Can you work these out from the model? Positions are in its coordinate system, mm. Coordinates: 2 decimals unless noted, no trailing zeros. Order: outer loops, then holes, each group sorted by start corner. A loop starts at its lowest first (then second) coordinate and runs counter-clockwise, first axis right, second up.
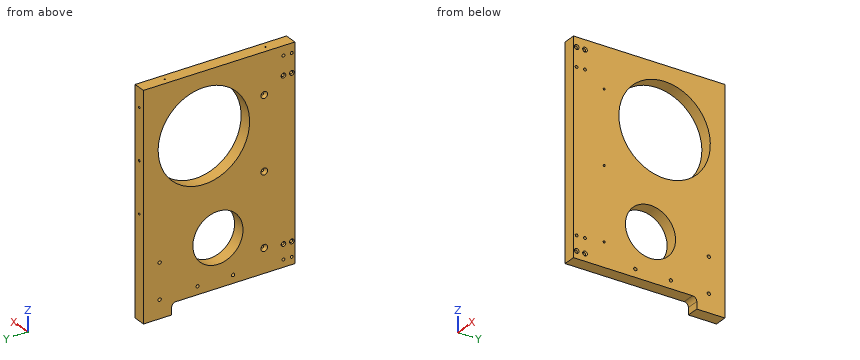
```python
from build123d import *

# Parameters (mm, degrees)
SKETCH1_W                                         = 19.05
SKETCH1_H                                         = 230.1875
BOSS_EXTRUDE1_DEPTH                               = 342.9
SKETCH2_W                                         = 19.05
SKETCH2_H                                         = 156.880836743
CUT_EXTRUDE1_DEPTH                                = 8.255
F_15_64_0_23438_DIAMETER_HOLE3_D                  = 5.953252
F_15_64_0_23438_DIAMETER_HOLE3_DEPTH              = 12.7
F_15_64_0_23438_DIAMETER_HOLE3_TIP                = 1.788537341
F_5_64_0_07813_DIAMETER_HOLE1_D                   = 3.175
F_5_64_0_07813_DIAMETER_HOLE1_DEPTH               = 38.1
F_5_64_0_07813_DIAMETER_HOLE1_CSINK_D             = 10.16
F_5_64_0_07813_DIAMETER_HOLE1_CSINK_ANGLE         = 82
F_5_64_0_07813_DIAMETER_HOLE1_TIP                 = 0.953866233
F_5_64_0_07813_DIAMETER_HOLE2_D                   = 1.984502
F_5_64_0_07813_DIAMETER_HOLE2_DEPTH               = 38.1
F_5_64_0_07813_DIAMETER_HOLE2_CSINK_D             = 10.16
F_5_64_0_07813_DIAMETER_HOLE2_CSINK_ANGLE         = 82
F_5_64_0_07813_DIAMETER_HOLE2_TIP                 = 0.59620455
F_1_8_0_125_DIAMETER_HOLE1_D                      = 3.175
F_1_8_0_125_DIAMETER_HOLE1_DEPTH                  = 19.05
F_1_8_0_125_DIAMETER_HOLE1_CSINK_D                = 10.16
F_1_8_0_125_DIAMETER_HOLE1_CSINK_ANGLE            = 90
F_8_CLEARANCE_HOLE1_D                             = 4.9149
F_8_CLEARANCE_HOLE1_DEPTH                         = 19.05
CSK_FOR_6_FLAT_HEAD_MACHINE_SCREW_100_D           = 4.3053
CSK_FOR_6_FLAT_HEAD_MACHINE_SCREW_100_DEPTH       = 19.05
CSK_FOR_6_FLAT_HEAD_MACHINE_SCREW_100_CSINK_D     = 7.0866
CSK_FOR_6_FLAT_HEAD_MACHINE_SCREW_100_CSINK_ANGLE = 82
CSK_FOR_6_FLAT_HEAD_MACHINE_SCREW1_D              = 4.3053
CSK_FOR_6_FLAT_HEAD_MACHINE_SCREW1_DEPTH          = 19.05
CSK_FOR_6_FLAT_HEAD_MACHINE_SCREW1_CSINK_D        = 7.0866
CSK_FOR_6_FLAT_HEAD_MACHINE_SCREW1_CSINK_ANGLE    = 82
CUT_EXTRUDE3_REACH                                = 21.05
SKETCH22_W                                        = 25.4
SKETCH22_H                                        = 187.3885
FILLET1_R                                         = 6.35
F_8_CLEARANCE_HOLE2_D                             = 4.9149
CUT_EXTRUDE2_REACH                                = 21.05
SKETCH17_R                                        = 69.5325
SKETCH17_R_2                                      = 38.1


with BuildPart() as part:
    # Sketch1 → Boss-Extrude1 (new body)
    with BuildSketch(Plane.XY):
        with Locations((-281.19705, -118.26875)):
            Rectangle(SKETCH1_W, SKETCH1_H)
    extrude(amount=BOSS_EXTRUDE1_DEPTH)

    # Sketch2 → Cut-Extrude1 (cut)
    with BuildSketch(Plane.XY):
        with Locations((-281.19705, -81.615418372)):
            Rectangle(SKETCH2_W, SKETCH2_H)
    extrude(amount=CUT_EXTRUDE1_DEPTH, mode=Mode.SUBTRACT)

    # 15/64 (0.23438) Diameter Hole3
    with Locations(Plane(origin=(-182.40375, 1936.853954382, -6.35), x_dir=(1, 0, 0), z_dir=(0, 0, -1))):
        with Locations((-262.8265, 2051.088542934), (-262.8265, 2014.068680083), (-262.8265, 1977.048817232), (-98.7933, 2115.959791125), (-98.7933, 2151.166454382)):
            Hole(F_15_64_0_23438_DIAMETER_HOLE3_D / 2, depth=F_15_64_0_23438_DIAMETER_HOLE3_DEPTH)
            with Locations((0, 0, -(F_15_64_0_23438_DIAMETER_HOLE3_DEPTH + F_15_64_0_23438_DIAMETER_HOLE3_TIP / 2))):  # 118° drill point
                Cone(0, F_15_64_0_23438_DIAMETER_HOLE3_D / 2, F_15_64_0_23438_DIAMETER_HOLE3_TIP, mode=Mode.SUBTRACT)

    # 5/64 (0.07813) Diameter Hole1
    with Locations(Plane(origin=(-182.40375, 15.875, 6471.459863233), x_dir=(1, 0, 0), z_dir=(0, 1, 0))):
        with Locations((-262.8265, 6157.452363233), (-98.7933, 6157.452363233), (-262.8265, 6233.652363233), (-98.7933, 6233.652363233), (-262.8265, 6309.852363233), (-98.7933, 6309.852363233), (-267.97, 6119.034863233), (-115.57, 6119.034863233), (-1.27, 6119.034863233), (113.03, 6119.034863233), (265.43, 6119.034863233), (96.2533, 6309.852363233), (260.2865, 6309.852363233), (96.2533, 6233.652363233), (260.2865, 6233.652363233), (96.2533, 6157.452363233), (260.2865, 6157.452363233)):
            CounterSinkHole(F_5_64_0_07813_DIAMETER_HOLE1_D / 2, F_5_64_0_07813_DIAMETER_HOLE1_CSINK_D / 2, depth=F_5_64_0_07813_DIAMETER_HOLE1_DEPTH, counter_sink_angle=F_5_64_0_07813_DIAMETER_HOLE1_CSINK_ANGLE)
            with Locations((0, 0, -(F_5_64_0_07813_DIAMETER_HOLE1_DEPTH + F_5_64_0_07813_DIAMETER_HOLE1_TIP / 2))):  # 118° drill point
                Cone(0, F_5_64_0_07813_DIAMETER_HOLE1_D / 2, F_5_64_0_07813_DIAMETER_HOLE1_TIP, mode=Mode.SUBTRACT)

    # 5/64 (0.07813) Diameter Hole2
    with Locations(Plane(origin=(-182.40375, 1936.853954382, 361.95), x_dir=(-1, 0, 0), z_dir=(0, 0, 1))):
        with Locations((-263.392416364, 1965.434682144), (262.8265, 1964.708862949), (262.8265, 2063.428497217), (98.7933, 2131.851871048), (98.7933, 1978.393537715), (53.56098, 2123.543954382), (-53.56098, 2123.543954382), (-99.322089753, 1978.666800322), (-98.898757225, 2132.124549748), (-263.120086856, 2064.153940785)):
            CounterSinkHole(F_5_64_0_07813_DIAMETER_HOLE2_D / 2, F_5_64_0_07813_DIAMETER_HOLE2_CSINK_D / 2, depth=F_5_64_0_07813_DIAMETER_HOLE2_DEPTH, counter_sink_angle=F_5_64_0_07813_DIAMETER_HOLE2_CSINK_ANGLE)
            with Locations((0, 0, -(F_5_64_0_07813_DIAMETER_HOLE2_DEPTH + F_5_64_0_07813_DIAMETER_HOLE2_TIP / 2))):  # 118° drill point
                Cone(0, F_5_64_0_07813_DIAMETER_HOLE2_D / 2, F_5_64_0_07813_DIAMETER_HOLE2_TIP, mode=Mode.SUBTRACT)

    # 1/8 (0.125) Diameter Hole1
    with Locations(Plane.ZY.offset(290.72205)):
        with Locations((61.9125, -186.69), (280.9875, -186.69), (171.45, -186.69)):
            CounterSinkHole(F_1_8_0_125_DIAMETER_HOLE1_D / 2, F_1_8_0_125_DIAMETER_HOLE1_CSINK_D / 2, depth=F_1_8_0_125_DIAMETER_HOLE1_DEPTH, counter_sink_angle=F_1_8_0_125_DIAMETER_HOLE1_CSINK_ANGLE)

    # #8 Clearance Hole1
    with Locations(Plane(origin=(-271.67205, 0, 0), x_dir=(0, 0, -1), z_dir=(1, 0, 0))):
        with Locations((-88.9, -27.7495), (-35.8275, -27.7495)):
            Hole(F_8_CLEARANCE_HOLE1_D / 2, depth=F_8_CLEARANCE_HOLE1_DEPTH)

    # CSK for #6 Flat Head Machine Screw (100)1
    with Locations(Plane(origin=(-271.67205, 0, 0), x_dir=(0, 0, -1), z_dir=(1, 0, 0))):
        with Locations((-36.5125, -215.9), (-36.5125, -228.6), (-328.6125, -215.9), (-328.6125, -228.6)):
            CounterSinkHole(CSK_FOR_6_FLAT_HEAD_MACHINE_SCREW_100_D / 2, CSK_FOR_6_FLAT_HEAD_MACHINE_SCREW_100_CSINK_D / 2, depth=CSK_FOR_6_FLAT_HEAD_MACHINE_SCREW_100_DEPTH, counter_sink_angle=CSK_FOR_6_FLAT_HEAD_MACHINE_SCREW_100_CSINK_ANGLE)

    # CSK for #6 Flat Head Machine Screw1
    with Locations(Plane.ZY.offset(290.72205)):
        with Locations((58.7375, -228.6), (58.7375, -215.9), (300.0375, -228.6), (300.0375, -215.9)):
            CounterSinkHole(CSK_FOR_6_FLAT_HEAD_MACHINE_SCREW1_D / 2, CSK_FOR_6_FLAT_HEAD_MACHINE_SCREW1_CSINK_D / 2, depth=CSK_FOR_6_FLAT_HEAD_MACHINE_SCREW1_DEPTH, counter_sink_angle=CSK_FOR_6_FLAT_HEAD_MACHINE_SCREW1_CSINK_ANGLE)

    # Sketch22 → Cut-Extrude3 (cut, up to next)
    with BuildSketch(Plane.ZY.offset(290.72205), mode=Mode.PRIVATE) as cut_extrude3_sk1:
        with Locations((12.7, -139.66825)):
            Rectangle(SKETCH22_W, SKETCH22_H)
    cut_extrude3_tool1 = extrude(cut_extrude3_sk1.sketch, amount=-CUT_EXTRUDE3_REACH, mode=Mode.PRIVATE) & part.part
    add(cut_extrude3_tool1.solids().sort_by_distance((-290.72205, -139.66825, 12.7))[0], mode=Mode.SUBTRACT)

    # Fillet1
    fillet1_edges = [part.edges().sort_by_distance(p)[0] for p in [
        (-281.19705, -45.974, 25.4),
    ]]
    fillet(fillet1_edges, radius=FILLET1_R)

    # #8 Clearance Hole2 (through all)
    with Locations(Plane(origin=(-271.67205, 0, 0), x_dir=(0, 0, -1), z_dir=(1, 0, 0))):
        with Locations((-37.44755, -139.371990921), (-37.44755, -85.396990921)):
            Hole(F_8_CLEARANCE_HOLE2_D / 2)

    # Sketch17 → Cut-Extrude2 (cut, up to next)
    with BuildSketch(Plane.ZY.offset(290.72205), mode=Mode.PRIVATE) as cut_extrude2_sk1:
        with Locations((250.03125, -94.9325)):
            Circle(SKETCH17_R)
    cut_extrude2_tool1 = extrude(cut_extrude2_sk1.sketch, amount=-CUT_EXTRUDE2_REACH, mode=Mode.PRIVATE) & part.part
    add(cut_extrude2_tool1.solids().sort_by_distance((-290.72205, -94.9325, 250.03125))[0], mode=Mode.SUBTRACT)
    # Sketch17 → Cut-Extrude2 (cut, up to next)
    with BuildSketch(Plane.ZY.offset(290.72205), mode=Mode.PRIVATE) as cut_extrude2_sk2:
        with Locations((97.63125, -116.332)):
            Circle(SKETCH17_R_2)
    cut_extrude2_tool2 = extrude(cut_extrude2_sk2.sketch, amount=-CUT_EXTRUDE2_REACH, mode=Mode.PRIVATE) & part.part
    add(cut_extrude2_tool2.solids().sort_by_distance((-290.72205, -116.332, 97.63125))[0], mode=Mode.SUBTRACT)


solid = part.part
```
1. Imagine slicing it at A-A on y = -100. Please give me the cut outline in (x, z).
Completed:
outline: (-290.72, 25.4) - (-271.67, 25.4) - (-271.67, 63.21) - (-290.72, 63.21) - close; (-290.72, 132.05) - (-271.67, 132.05) - (-271.67, 180.68) - (-290.72, 180.68) - close; (-290.72, 319.38) - (-271.67, 319.38) - (-271.67, 342.9) - (-290.72, 342.9) - close
2. Imagine slicing it at B-B on z = 195. Please give me the cut outline in (x, y) (1 decimal).
Completed:
outline: (-290.7, -233.4) - (-271.7, -233.4) - (-271.7, -137.4) - (-290.7, -137.4) - close; (-290.7, -52.4) - (-271.7, -52.4) - (-271.7, -3.2) - (-290.7, -3.2) - close
3. I'm going to push flat-ended pins straight in: pin 1 (5 mm diameter, centred on y = -186.69, z = 171.45, fed in from -X); pin 2 (4 mm diameter, centred on y = -215.9, z = 58.74, fed in from -X); pin 3 (9.5 mm diameter, centred on x = -284.5, y = -134.5, fed in from -Z); pin 4 (5.5 mm diameter, centred on y = -228.6, z = 36.51, fed in from +X). Where does each tip first touch, or does it pass through?
Completed:
pin 1: stops at x = -288.14
pin 2: passes through
pin 3: stops at z = 25.4
pin 4: stops at x = -272.58
4. Please list where these lines run through material, in increasing order: probe 1 along Z at (x, y) = (-281, -228.6); probe 2 along Z at (x, y) = (-272.5, -114.5); probe 3 along Y at (x, z) = (-275.75, 37) (1 decimal).
Completed:
probe 1: z = 25.4 to 34.36, 38.67 to 56.58, 60.89 to 297.88, 302.19 to 326.46, 330.77 to 342.9
probe 2: z = 25.4 to 59.58, 135.69 to 183.31, 316.75 to 342.9
probe 3: y = -233.4 to -230.7, -226.5 to -218, -213.8 to -141.8, -137 to -87.8, -83 to -29.9, -25.6 to -3.2
